from build123d import *

# Parameters (mm, degrees)
F0_R     = 37.5
F0_R_2   = 1.500821
F1_DEPTH = 11


with BuildPart() as f1:
    # F0 (on Front) → F1 (new body)
    with BuildSketch(Plane.XZ):
        Circle(F0_R)
        with BuildLine():
            Line((-28.472292, -2.5), (-15.499999, -2.500001))
            ThreePointArc((-15.499999, -2.500001), (-6.307613, -6.307613), (-2.500001, -15.499999))
            Line((-2.500001, -15.499999), (-2.500189, -28.5))
            Line((-2.500189, -28.5), (-11.805087, -28.5))
            Line((-11.805087, -28.5), (-28.5, -11.805087))
            Line((-28.5, -11.805087), (-28.472292, -2.5))
        make_face(mode=Mode.SUBTRACT)
        with BuildLine():
            ThreePointArc((2.500001, -15.499999), (6.307613, -6.307612), (15.500001, -2.5))
            Line((15.500001, -2.5), (28.5, -2.5))
            Line((28.5, -2.5), (28.5, -11.805087))
            Line((28.5, -11.805087), (11.805087, -28.5))
            Line((11.805087, -28.5), (2.500189, -28.5))
            Line((2.500189, -28.5), (2.500001, -15.499999))
        make_face(mode=Mode.SUBTRACT)
        with BuildLine():
            ThreePointArc((-2.499999, 15.500001), (-6.307611, 6.307612), (-15.499999, 2.5))
            Line((-15.499999, 2.5), (-28.472292, 2.5))
            Line((-28.472292, 2.5), (-28.5, 11.805087))
            Line((-28.5, 11.805087), (-11.805087, 28.5))
            Line((-11.805087, 28.5), (-2.499811, 28.5))
            Line((-2.499811, 28.5), (-2.499999, 15.500001))
        make_face(mode=Mode.SUBTRACT)
        Circle(F0_R_2, mode=Mode.SUBTRACT)
        with BuildLine():
            Line((28.5, 2.5), (15.500001, 2.5))
            ThreePointArc((15.500001, 2.5), (6.307612, 6.307612), (2.5, 15.500001))
            Line((2.5, 15.500001), (2.499811, 28.5))
            Line((2.499811, 28.5), (11.805087, 28.5))
            Line((11.805087, 28.5), (28.5, 11.805087))
            Line((28.5, 11.805087), (28.5, 2.5))
        make_face(mode=Mode.SUBTRACT)
    extrude(amount=F1_DEPTH)


solid = f1.part
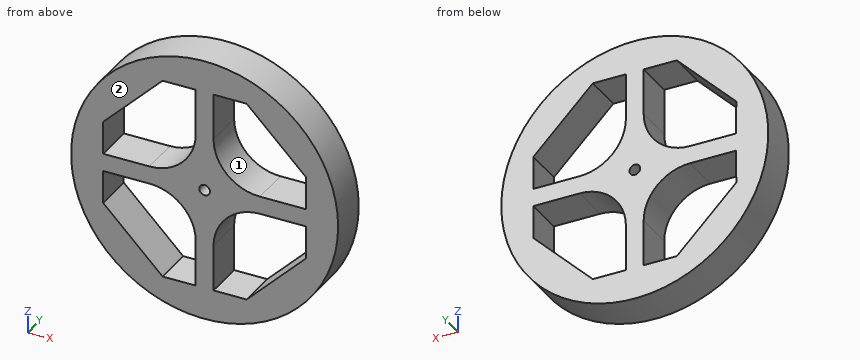
Design review of the part built by this model. Coordinates are the model's own, in mm. Face numbers are marked on the shaded views. Round coordinates to 2 decimals unless told otherwise and drop trailing zeros. Write each loop counter-clockwise with the first axis right and the second up, starting at its lowest first coordinate (ties: lowest second). Pieces come first, ordered by that corner, then holes. Notation, with made-up numbers: (18, 22.25) - (77, 22.25) arc R14 cw to (77, 45.25) - close; hole circle Ø9 at (13.25, 40.5). An arc over 180 degrees is marked (long way). Use a Markdown table: item, result. Add a question column.
1. We need section D-D (x = -26). State the section outline as (y, z) points.
2. We need section C-C (z = 0). State the section outline as (x, y) points, then the cut area to 3 significant figures.
3. Wall thickness on probe 1 along X at (y, z) = (-3.5, -14.5); probe 2 along X at (y, z) = (-8.25, 27); probe 3 along Z at (x, y) = (-14, -0.75): over which ranges is each line inside the solid? List them lowest first.
4. We need section A-A (x = 0). State the section outline as (y, z) points, then the cut area to 3 significant figures.
5. Mouldability with a two-part tool opening along Z and no side actions: class the marked faces 1 and 2 as +Z half, -Z half, draft (parallel to the pull), parting line (faces both ways), or undercut.
6. Clearance check with flat-ended pins moving along their axes: pin 1 (4.5 mm diameter, centred on x = 5, y = -7, fed in from +Z); pin 2 (5 mm diameter, centred on y = -9.5, z = 26.5, fed in from -X); pin 3 (4.5 mm diameter, centred on y = -5.5, z = -8, fed in from -X). State where each tip first meets the part, or that it passes through.
7. We need section B-B (y = -1.5). State the section outline as (x, z) points, then the cut area to 3 significant figures.
Output:
| question | item | result |
|---|---|---|
| 1 | outline | (-11, -27.02) - (0, -27.02) - (0, -14.31) - (-11, -14.31) - close; (-11, -2.5) - (0, -2.5) - (0, 2.5) - (-11, 2.5) - close; (-11, 14.31) - (0, 14.31) - (0, 27.02) - (-11, 27.02) - close |
| 2 | outline | (-37.5, -11) - (-1.5, -11) - (-1.5, 0) - (-37.5, 0) - close; (1.5, -11) - (37.5, -11) - (37.5, 0) - (1.5, 0) - close |
| 2 | area | 792 mm2 |
| 3 | probe 1 | x = -34.58 to -25.81, -2.54 to 2.54, 25.81 to 34.58 |
| 3 | probe 2 | x = -26.02 to -13.31, -2.5 to 2.5, 13.31 to 26.02 |
| 3 | probe 3 | z = -34.79 to -26.31, -2.59 to 2.59, 26.31 to 34.79 |
| 4 | outline | (-11, -37.5) - (0, -37.5) - (0, -1.5) - (-11, -1.5) - close; (-11, 1.5) - (0, 1.5) - (0, 37.5) - (-11, 37.5) - close |
| 4 | area | 792 mm2 |
| 5 | face 1 | undercut |
| 5 | face 2 | draft |
| 6 | pin 1 | stops at z = 37.4 |
| 6 | pin 2 | stops at x = -28.81 |
| 6 | pin 3 | stops at x = -37.06 |
| 7 | outline | circle Ø75 at (0, 0); hole (-28.5, -11.81) - (-11.81, -28.5) - (-2.5, -28.5) - (-2.5, -15.5) arc R13 ccw to (-15.5, -2.5) - (-28.47, -2.5) - close; hole (-28.5, 11.81) - (-28.47, 2.5) - (-15.5, 2.5) arc R13 ccw to (-2.5, 15.5) - (-2.5, 28.5) - (-11.81, 28.5) - close; hole circle Ø3 at (0, 0); hole (2.5, -28.5) - (11.81, -28.5) - (28.5, -11.81) - (28.5, -2.5) - (15.5, -2.5) arc R13 ccw to (2.5, -15.5) - close; hole (2.5, 15.5) arc R13 ccw to (15.5, 2.5) - (28.5, 2.5) - (28.5, 11.81) - (11.81, 28.5) - (2.5, 28.5) - close |
| 7 | area | 2,410 mm2 |
